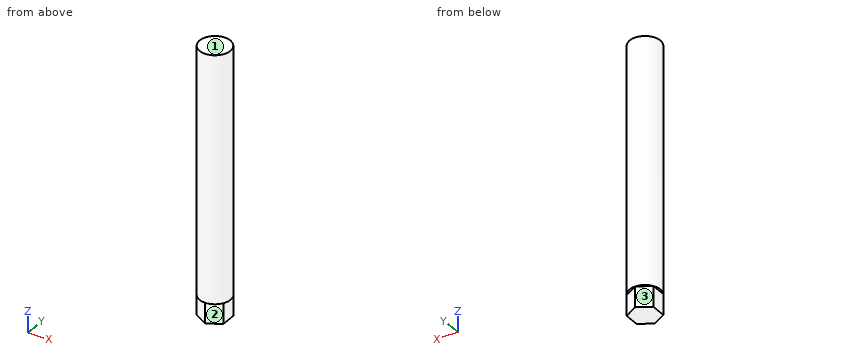
Autodesk Inventor part; units mm, degrees
ref_plane "YZ Plane" through (0, 0, 0) normal (1, 0, 0) x (0, 1, 0)
ref_plane "XZ Plane" through (0, 0, 0) normal (0, 1, 0) x (-1, 0, 0)
ref_plane "XY Plane" through (0, 0, 0) normal (0, 0, 1) x (1, 0, 0)
sketch "Szkic1" plane through (0, 0, 0) normal (0, 0, 1) x (1, 0, 0)
  circle A0 centre (-4.3569, 3.3954) radius 15
  point P0 (0, 0)
  dimension "d0" = 30
extrude "Wyciągnięcie proste1" add sketch "Szkic1" along normal blind 240
thread "Gwint1"
thread "Gwint2"
sketch "Szkic2" plane through (-4.3569, 3.3954, 0) normal (0, 0, -1) x (-1, 0, 0)
  circle A0 centre (0, 0) radius 15
  line L0 (0, 15) -> (12.9904, 7.5)
  line L1 (12.9904, 7.5) -> (12.9904, -7.5)
  line L2 (12.9904, -7.5) -> (0, -15)
  line L3 (0, -15) -> (-12.9904, -7.5)
  line L4 (-12.9904, -7.5) -> (-12.9904, 7.5)
  line L5 (-12.9904, 7.5) -> (0, 15)
  point P0 (-4.3569, -3.3954)
  dimension "d9" = 360
extrude "Wyciągnięcie proste2" add sketch "Szkic2" along normal blind 20 contours L1 L2 L3 L4 L5 L0
properties part number "śruba"
Geometry: final body of the model. Coordinates: model frame, mm. Face numbers are marked on the shaded views. A direction names the side the tool comes from. Round coordinates to 2 decimals unless told otherwise and drop trailing zeros. Order: outer loops, then holes, each group sorted by start corner. A loop starts at its lowest first (then second) coordinate and runs counter-clockwise, first axis right, second up. Notation, with made-up numbers: (-3.75, -37.75) -> (53.25, -37.75) arc R14 cw to (53.25, -25.75) -> close; hole circle Ø9 at (79, 30.25). An arc over 180 degrees is marked (long way). Put each result on its own line as item: value. Start each with the question number.
Q1. Reachability of the marked faces 1, 2 and 3 from +Z, -Z, +X, -X, +Y, -Y: full face, straight path, thin tool, end or side. Return the list, or none.
Q2. Section C-C on z = 139.5. Return the cut outline in (x, y), and give its area (3 significant figures).
Q3. Section B-B on x = -13. Return the cut outline in (y, z), and give its area (4 significant figures).
Q4. Section A-A on y = 15.5. Return the cut outline in (x, z), and give its area (3 significant figures).
Q5. First-contact query: pin 1 (4 mm diameter, centred on x = 6, z = 14.5, fed in from -Y); pin 2 (1 mm diameter, centred on x = -1.5, z = 41, fed in from +Y); pin 3 (3 mm diameter, centred on y = 14, z = 139.5, fed in from -X). Flat tips, straight axial feed; report the tip coordinate or a pass-through.
Q6. Line query: probe 1 along Y at (x, z) = (-3.5, 140); probe 2 along X at (y, z) = (3, 186); probe 3 along X at (y, z) = (2.5, 122.5). Output: solid intervals per line, ascending.
Ans:
1. face 1: +Z, +X, -X, +Y, -Y
1. face 2: -Z, +X, -Y
1. face 3: -Z, -X, +Y
2. outline: circle Ø30 at (-4.36, 3.4)
2. area: 707 mm2
3. outline: (-8.86, 0) -> (-6.61, 0) -> (-6.61, -20) -> (13.41, -20) -> (13.41, 0) -> (15.65, 0) -> (15.65, 240) -> (-8.86, 240) -> close
3. area: 6,285 mm2
4. outline: (-13.22, 0) -> (-9.37, 0) -> (-9.37, -20) -> (0.66, -20) -> (0.66, 0) -> (4.5, 0) -> (4.5, 240) -> (-13.22, 240) -> close
4. area: 4,450 mm2
5. pin 1: stops at y = -9.06
5. pin 2: stops at y = 18.21
5. pin 3: stops at x = -16.28
6. probe 1: y = -11.58 to 18.37
6. probe 2: x = -19.35 to 10.64
6. probe 3: x = -19.33 to 10.62
